For this review, use the dimensioned drawing (mm, ordinates from the lowest corner) and the shaded views. Give positions to 0.01 mm unless a question says otherwise; leave off trailing zeros. Write each loop counter-clockwise with the first axis right and the second up, starting at its lowest first coordinate (ties: lowest second). Pieces come first, ordered by that corner, then holes. Notation, with made-up numbers: (37.5, -26.5) -> (90.5, -26.5) arc R20 cw to (90.5, 6.5) -> close; hole circle Ø4 at (63.25, -19.5). An arc over 180 degrees is marked (long way). Answer as CSV lines item,"result".
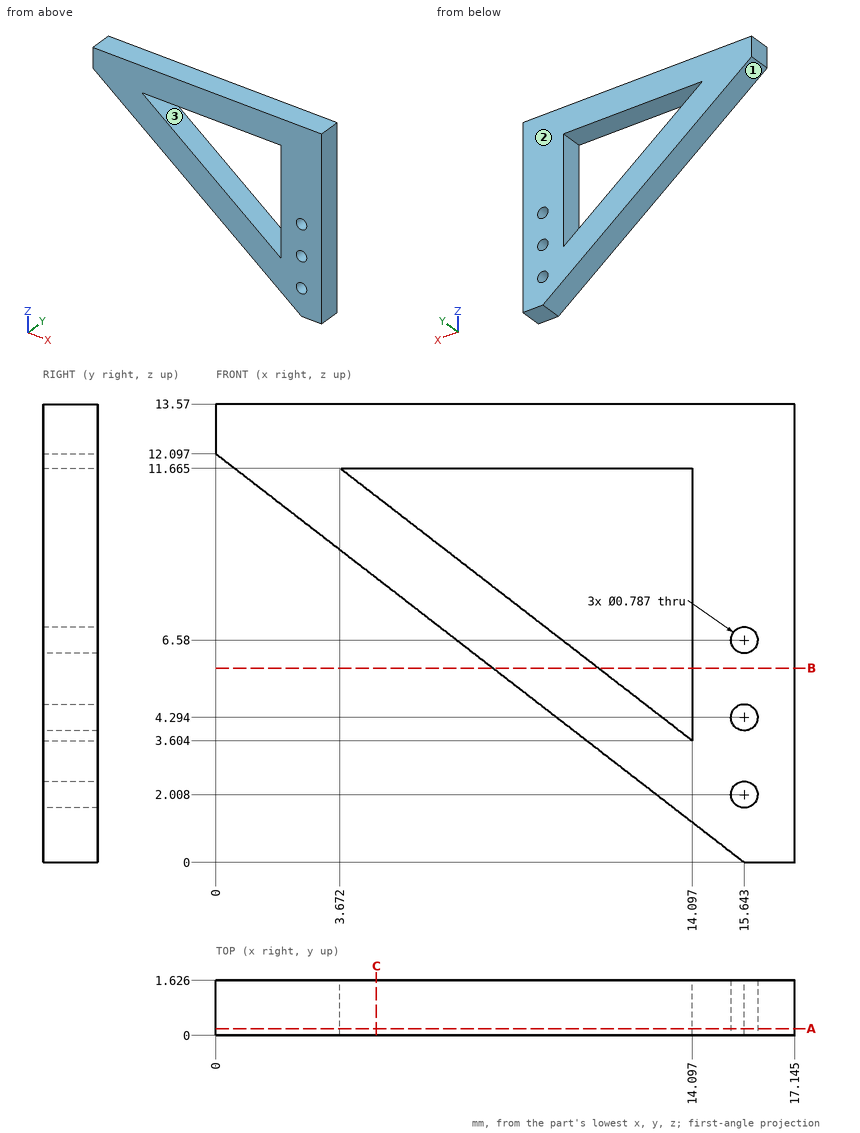
Q1. Add section B-B (z = 5.75). Write out the cut boundary in (x, y) (1 decimal).
Answer block:
outline,"(8.2, 0) -> (11.3, 0) -> (11.3, 1.6) -> (8.2, 1.6) -> close; (14.1, 0) -> (17.1, 0) -> (17.1, 1.6) -> (14.1, 1.6) -> close"
Q2. Add section A-A (y = 0.2). Write out the cut boundary in (x, z) (1 decimal).
Answer block:
outline,"(0, 12.1) -> (15.6, 0) -> (17.1, 0) -> (17.1, 13.6) -> (0, 13.6) -> close; hole (3.7, 11.7) -> (14.1, 3.6) -> (14.1, 11.7) -> close; hole circle Ø0.8 at (15.6, 2); hole circle Ø0.8 at (15.6, 4.3); hole circle Ø0.8 at (15.6, 6.6)"
Q3. Clearance check with flat-ended pins moving along their axes: pin 1 (0.8 mm diameter, centred on y = 0.5, z = 7, fed in from -X) (1 decimal); pin 2 (0.5 mm diameter, centred on x = 10, y = 1, fed in from -Z). State where each tip first meets the part, or that it passes through.
Answer block:
pin 1,"stops at x = 6.1"
pin 2,"stops at z = 4.17"
Q4. Draft analysis for pull direction Z (two halves, no side actions). For the marked faces 1, 2 and 3, state which applies: released by +Z, released by -Z, zero draft, split by the parting line, or undercut.
Answer block:
face 1,"released by -Z"
face 2,"zero draft"
face 3,"undercut"
Q5. Add section C-C (x = 4.75). Write out the cut boundary in (y, z) (1 decimal).
Answer block:
outline,"(0, 8.4) -> (1.6, 8.4) -> (1.6, 10.8) -> (0, 10.8) -> close; (0, 11.7) -> (1.6, 11.7) -> (1.6, 13.6) -> (0, 13.6) -> close"
Q6. To check wall thickness, follow probe 1 along X at (y, z) = (1.55, 6.75) (1 decimal); probe 2 along Z at (x, y) = (15.75, 1.25) (1 decimal); probe 3 along X at (y, z) = (0.3, 4.5) (1 decimal). State the ranges of each line that lie inside material, in increasing order. Write a range as [from, to].
Answer block:
probe 1,"x = [6.9, 10], [14.1, 15.3], [16, 17.1]"
probe 2,"z = [0, 1.6], [2.4, 3.9], [4.7, 6.2], [7, 13.6]"
probe 3,"x = [9.8, 12.9], [14.1, 15.3], [16, 17.1]"
